Geometry: see drawing. Coordinates: mm, zero at the bounding-box minimum. A direction names the side the tool comes from. Coordinates: 2 decimals unless noted, no trailing zeros. Write each loop counter-clockwise with the first axis right and the second up, starting at its lowest first coordinate (ties: lowest second). Pieces come first, ordered by that corner, then holes. Notation, with made-up numbers: (75, -37) - (88, -37) arc R19 ccw to (88, -12) - close; hole circle Ø7 at (21, 55). An arc over 180 degrees is marked (long way). Use CSV: the item, a comma, the result in double quotes.
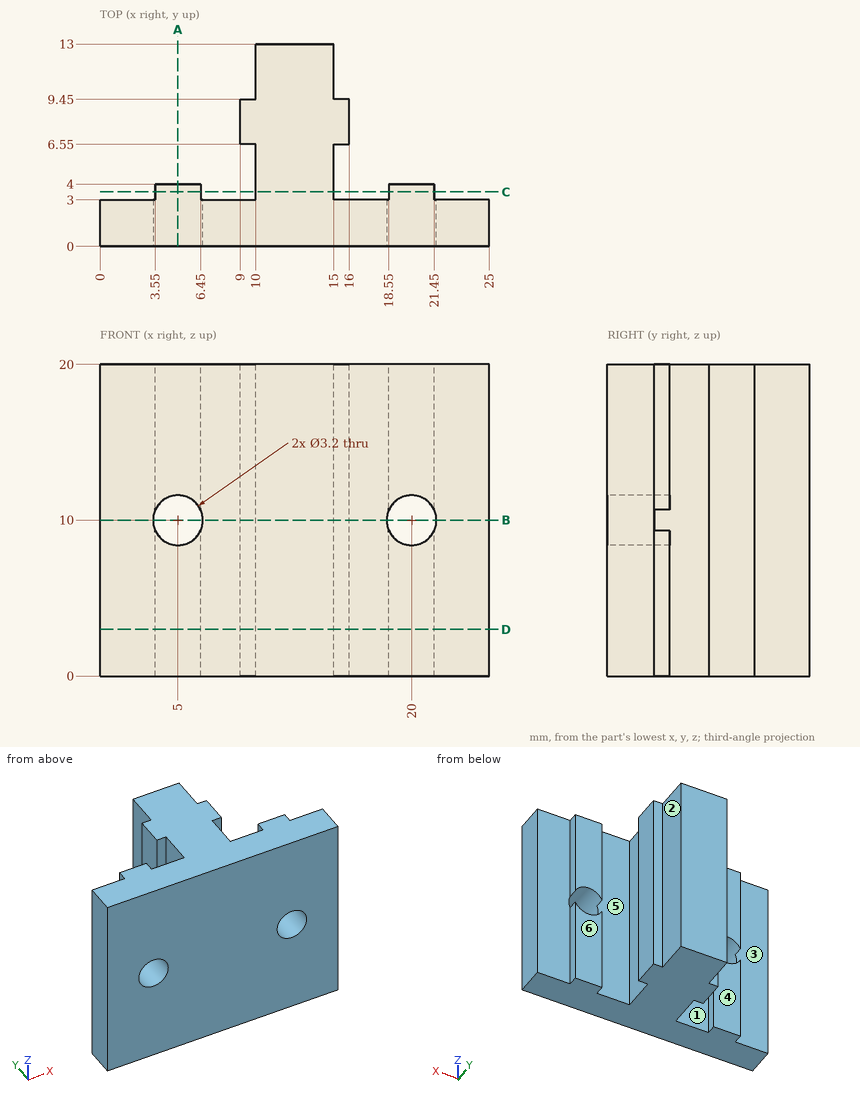
(1) Reachability of the marked faces 4, 5 and 6 from +Z, -Z, +X, -X, +Y, -Y: full face, straight path, thin tool, end or side. Return the list, or none.
Check values:
face 4,"+Z, -Z, -X, +Y"
face 5,"+Z, -Z"
face 6,"+Z, -Z, +X, +Y"
(2) Cut plane D-D on z = 3. Return loops of the section in (x, y).
Check values:
outline,"(0, 0) - (25, 0) - (25, 3) - (21.45, 3) - (21.45, 4) - (18.55, 4) - (18.55, 3) - (15, 3) - (15, 6.55) - (16, 6.55) - (16, 9.45) - (15, 9.45) - (15, 13) - (10, 13) - (10, 9.45) - (9, 9.45) - (9, 6.55) - (10, 6.55) - (10, 3) - (6.45, 3) - (6.45, 4) - (3.55, 4) - (3.55, 3) - (0, 3) - close"
(3) Cut plane A-A on x = 5. Return loops of the section in (y, z).
Check values:
outline,"(0, 0) - (4, 0) - (4, 8.4) - (0, 8.4) - close; (0, 11.6) - (4, 11.6) - (4, 20) - (0, 20) - close"
(4) Pin query (flat end, axial travel): pin 1 Ø3 at (x, z) = (20.5, 2.5) entering from +Y; pin 2 Ø1 at (y, z) = (11.5, 18) entering from +X; pin 3 Ø1.5 at (y, z) = (5, 12) entering from -X. Return the tip coordinate at first contact, or that it passes through.
Check values:
pin 1,"y = 4"
pin 2,"x = 15"
pin 3,"x = 10"
(5) Ray query, probe 1 along Z at (x, y) = (5, 2.2); probe 2 along Y at (x, z) = (9.25, 8.75); probe 3 along Y at (x, z) = (5.75, 19). Return the intervals inside material, ascending. Write a range as from..to.
Check values:
probe 1,"0..8.4, 11.6..20"
probe 2,"0..3, 6.55..9.45"
probe 3,"0..4"
(6) Cut plane C-C on y = 3.5. Return loops of the section in (x, z), and give its area (3 significant figures).
Check values:
outline,"(3.55, 0) - (6.45, 0) - (6.45, 9.32) arc R1.6 cw to (3.55, 9.32) - close; (3.55, 10.68) arc R1.6 cw to (6.45, 10.68) - (6.45, 20) - (3.55, 20) - close; (10, 0) - (15, 0) - (15, 20) - (10, 20) - close; (18.55, 0) - (21.45, 0) - (21.45, 9.32) arc R1.6 cw to (18.55, 9.32) - close; (18.55, 10.68) arc R1.6 cw to (21.45, 10.68) - (21.45, 20) - (18.55, 20) - close"
area,"200 mm^2"
(7) Draft query along X for the marked faces 1, 2 and 3. Return one class per face: pulls with the +X half, pulls with the -X half, needs draft (parallel to the pull), parting line crosses it, or undercut.
Check values:
face 1,"undercut"
face 2,"pulls with the +X half"
face 3,"needs draft"
(8) Cut plane B-B on z = 10. Return loops of the section in (x, y), and give its area (3 significant figures).
Check values:
outline,"(0, 0) - (3.4, 0) - (3.4, 3) - (0, 3) - close; (6.6, 0) - (18.4, 0) - (18.4, 3) - (15, 3) - (15, 6.55) - (16, 6.55) - (16, 9.45) - (15, 9.45) - (15, 13) - (10, 13) - (10, 9.45) - (9, 9.45) - (9, 6.55) - (10, 6.55) - (10, 3) - (6.6, 3) - close; (21.6, 0) - (25, 0) - (25, 3) - (21.6, 3) - close"
area,"112 mm^2"
